Can you work these out from the model? Positions are in its coordinate system, mm. Coordinates: 2 decimals unless noted, no trailing zeros. Loops run counter-clockwise (first coordinate to the right, second up) from the corner with the lowest first, then second, coordinate; pieces in that order, holes last.
```python
from build123d import *

# Parameters (mm, degrees)
F0_R     = 3.2639
F1_DEPTH = 4.7752


with BuildPart() as f1:
    # F0 (on Top) → F1 (new body)
    with BuildSketch(Plane.XY):
        Polygon((25.4, -12.70551), (12.7, 38.10551), (-12.7, 38.10551), (-25.402755, -12.70551), (-25.402755, -38.10551), (25.4, -38.10551), align=None)
        with Locations((-12.702755, -25.40551)):
            Circle(F0_R, mode=Mode.SUBTRACT)
        with Locations((12.702755, -25.40551)):
            Circle(F0_R, mode=Mode.SUBTRACT)
        Circle(F0_R, mode=Mode.SUBTRACT)
        with Locations((0, 25.40551)):
            Circle(F0_R, mode=Mode.SUBTRACT)
    extrude(amount=F1_DEPTH)


solid = f1.part
```
Item 1: Suppose I cut it at B-B, the plane y = 0. Please give me the cut outline in (x, z).
Results are:
outline: (-22.23, 0) - (-3.26, 0) - (-3.26, 4.78) - (-22.23, 4.78) - close; (3.26, 0) - (22.22, 0) - (22.22, 4.78) - (3.26, 4.78) - close
Item 2: We'd pull the mould along Y, two halves only. Please class faces 1 (the face through (19.14, 12.34, 2.35)), 2 (the face through (-0.71, 22.22, 2.35)), 3 (the face through (0, -8, 4.775)), 4 (the face through (-11.197, -28.301, 2.354)): +Y half, -Y half, draft (parallel to the pull), parting line (faces both ways), or undercut.
Results are:
face 1: +Y half
face 2: undercut
face 3: draft
face 4: undercut
Item 3: Suppose I cut it at D-D, the plane x = -13.5. Please give me the cut outline in (y, z).
Results are:
outline: (-38.11, 0) - (-28.57, 0) - (-28.57, 4.78) - (-38.11, 4.78) - close; (-22.24, 0) - (34.91, 0) - (34.91, 4.78) - (-22.24, 4.78) - close
Item 4: I'm going to push flat-ended pins straight in: P1, Ø1, axis at x = 10.5, y = 12, coming from the -Z side; P2, Ø5, axis at x = 0, y = 0, coming from the +Z side. Where does each tip first touch, or does it pass through?
Results are:
P1: stops at z = 0
P2: passes through
Item 5: Suppose I cut it at A-A, the plane x = 0. Please give me the cut outline in (y, z), plus the area to 3 significant figures.
Results are:
outline: (-38.11, 0) - (-3.26, 0) - (-3.26, 4.78) - (-38.11, 4.78) - close; (3.26, 0) - (22.14, 0) - (22.14, 4.78) - (3.26, 4.78) - close; (28.67, 0) - (38.11, 0) - (38.11, 4.78) - (28.67, 4.78) - close
area: 302 mm2
Item 6: I need wall thicknesses on line 1 along Y through (x, z) = (0, 2.35); line 2 along Y through (x, z) = (0.5, 3.4); line 3 along Y through (x, z) = (-12.5, 1.7). Which ranges of each line are inside material? Lowest first, please.
Results are:
line 1: y = -38.11 to -3.26, 3.26 to 22.14, 28.67 to 38.11
line 2: y = -38.11 to -3.23, 3.23 to 22.18, 28.63 to 38.11
line 3: y = -38.11 to -28.66, -22.15 to 38.11
Item 7: Suppose I cut it at C-C, the plane z = 2.8. Please give me the cut outline in (x, y).
Results are:
outline: (-25.4, -38.11) - (25.4, -38.11) - (25.4, -12.71) - (12.7, 38.11) - (-12.7, 38.11) - (-25.4, -12.71) - close; hole circle Ø6.53 at (-12.7, -25.41); hole circle Ø6.53 at (0, 0); hole circle Ø6.53 at (0, 25.41); hole circle Ø6.53 at (12.7, -25.41)
